from build123d import *

# Parameters (mm, degrees)
CROQUIS1_W                        = 25
CROQUIS1_H                        = 12.5
CROQUIS2_R                        = 3.5
SALIENTE_EXTRUIR1_DEPTH           = 2.5
CROQUIS3_R                        = 1.75
SALIENTE_EXTRUIR2_DEPTH           = 9.5
CORTAR_EXTRUIR1_DEPTH             = 8
CROQUIS5_R                        = 12.2
SALIENTE_EXTRUIR3_DEPTH           = 18
DI_METRO_DE_TALADRO_3_0_3_1_D     = 3
DI_METRO_DE_TALADRO_3_0_3_1_DEPTH = 8
CROQUIS10_R                       = 11.5
CORTAR_EXTRUIR2_DEPTH             = 2
SALIENTE_EXTRUIR4_DEPTH           = 1
CROQUIS12_W                       = 0.4
CROQUIS12_H                       = 3
SALIENTE_EXTRUIR5_DEPTH           = 6
REDONDEO1_R                       = 1
CORTAR_EXTRUIR3_DEPTH             = 57.252161552
CROQUIS15_R                       = 2.5
SALIENTE_EXTRUIR6_DEPTH           = 2
CROQUIS16_R                       = 1.5
SALIENTE_EXTRUIR7_DEPTH           = 3
CHAFL_N1_SIZE2                    = 0.363970234
CHAFL_N1_SIZE                     = 1
CROQUIS17_R                       = 1
CORTAR_EXTRUIR4_DEPTH             = 1


with BuildPart() as part:
    # Croquis1 → Revolución1 (revolve)
    with BuildSketch(Plane(origin=(0, 0, 0), x_dir=(-1, 0, 0), z_dir=(0, 0, -1)), mode=Mode.PRIVATE) as revoluci_n1_sk:
        with Locations((14, 12.15)):
            Rectangle(CROQUIS1_W, CROQUIS1_H)
    revolve(revoluci_n1_sk.sketch.rotate(Axis((-1.5, 5.9, 0), (-1, 0, 0)), 270), axis=Axis((-1.5, 5.9, 0), (-1, 0, 0)))

    # Croquis2 → Saliente-Extruir1 (add)
    with BuildSketch(Plane(origin=(-1.5, 0, 0), x_dir=(0, 0, -1), z_dir=(1, 0, 0))):
        with Locations((0, 5.9)):
            Circle(CROQUIS2_R)
    extrude(amount=SALIENTE_EXTRUIR1_DEPTH)

    # Croquis3 → Saliente-Extruir2 (add)
    with BuildSketch(Plane(origin=(1, 0, 0), x_dir=(0, 0, -1), z_dir=(1, 0, 0))):
        with Locations((0, 5.9)):
            Circle(CROQUIS3_R)
    extrude(amount=SALIENTE_EXTRUIR2_DEPTH)

    # Croquis4 → Cortar-Extruir1 (cut)
    with BuildSketch(Plane(origin=(10.5, 0, 0), x_dir=(0, 0, -1), z_dir=(1, 0, 0))):
        with BuildLine():
            Line((-1.496663044, 4.15), (1.496663044, 4.15))
            ThreePointArc((1.496663044, 4.15), (0, 4.264202971), (-1.496663044, 4.15))
        make_face()
    extrude(amount=-CORTAR_EXTRUIR1_DEPTH, mode=Mode.SUBTRACT)

    # Croquis5 → Saliente-Extruir3 (add)
    with BuildSketch(Plane.ZY.offset(26.5)):
        with Locations((0, 5.9)):
            Circle(CROQUIS5_R)
    extrude(amount=SALIENTE_EXTRUIR3_DEPTH)

    # Diámetro de taladro Ø3.0 (3)1
    with Locations(Plane(origin=(-1.5, 0, 0), x_dir=(0, 0, -1), z_dir=(1, 0, 0))):
        with Locations((-8.5, 5.827133015), (8.5, 5.827133015)):
            Hole(DI_METRO_DE_TALADRO_3_0_3_1_D / 2, depth=DI_METRO_DE_TALADRO_3_0_3_1_DEPTH)

    # Croquis10 → Cortar-Extruir2 (cut)
    with BuildSketch(Plane.ZY.offset(44.5)):
        with Locations((0, 5.9)):
            Circle(CROQUIS10_R)
    extrude(amount=-CORTAR_EXTRUIR2_DEPTH, mode=Mode.SUBTRACT)

    # Croquis11 → Saliente-Extruir4 (add)
    with BuildSketch(Plane.ZY.offset(42.5)):
        with BuildLine():
            Line((-5.135046812, 3.4), (-6.135046812, 3.4))
            ThreePointArc((-6.135046812, 3.4), (-6.488600202, 3.546446609), (-6.635046812, 3.9))
            Line((-6.635046812, 3.9), (-6.635046812, 7.9))
            ThreePointArc((-6.635046812, 7.9), (-6.488600202, 8.253553391), (-6.135046812, 8.4))
            Line((-6.135046812, 8.4), (-5.135046812, 8.4))
            ThreePointArc((-5.135046812, 8.4), (-4.781493421, 8.253553391), (-4.635046812, 7.9))
            Line((-4.635046812, 7.9), (-4.635046812, 3.9))
            ThreePointArc((-4.635046812, 3.9), (-4.781493421, 3.546446609), (-5.135046812, 3.4))
        make_face()
        with BuildLine():
            Line((7.124953188, 3.4), (6.124953188, 3.4))
            ThreePointArc((6.124953188, 3.4), (5.771399798, 3.546446609), (5.624953188, 3.9))
            Line((5.624953188, 3.9), (5.624953188, 7.9))
            ThreePointArc((5.624953188, 7.9), (5.771399798, 8.253553391), (6.124953188, 8.4))
            Line((6.124953188, 8.4), (7.124953188, 8.4))
            ThreePointArc((7.124953188, 8.4), (7.478506579, 8.253553391), (7.624953188, 7.9))
            Line((7.624953188, 7.9), (7.624953188, 3.9))
            ThreePointArc((7.624953188, 3.9), (7.478506579, 3.546446609), (7.124953188, 3.4))
        make_face()
    extrude(amount=SALIENTE_EXTRUIR4_DEPTH)

    # Croquis12 → Saliente-Extruir5 (add)
    with BuildSketch(Plane.ZY.offset(43.5)):
        with Locations((-5.637636684, 5.837666005)):
            Rectangle(CROQUIS12_W, CROQUIS12_H)
        with Locations((6.677710889, 5.9)):
            Rectangle(CROQUIS12_W, CROQUIS12_H)
    extrude(amount=SALIENTE_EXTRUIR5_DEPTH)

    # Redondeo1
    redondeo1_edges = [part.edges().sort_by_distance(p)[0] for p in [
        (-49.5, 4.337666005, -5.637636684),
        (-49.5, 7.337666005, -5.637636684),
        (-49.5, 4.4, 6.677710889),
        (-49.5, 7.4, 6.677710889),
    ]]
    fillet(redondeo1_edges, radius=REDONDEO1_R)

    # Croquis14 → Cortar-Extruir3 (cut, through all)
    with BuildSketch(Plane.XY.offset(6.877710889)):
        with BuildLine():
            Line((-45.3, 5.2), (-47.7, 5.2))
            ThreePointArc((-47.7, 5.2), (-47.912132034, 5.287867966), (-48, 5.5))
            Line((-48, 5.5), (-48, 6.3))
            ThreePointArc((-48, 6.3), (-47.912132034, 6.512132034), (-47.7, 6.6))
            Line((-47.7, 6.6), (-45.3, 6.6))
            ThreePointArc((-45.3, 6.6), (-45.087867966, 6.512132034), (-45, 6.3))
            Line((-45, 6.3), (-45, 5.5))
            ThreePointArc((-45, 5.5), (-45.087867966, 5.287867966), (-45.3, 5.2))
        make_face()
    extrude(amount=-CORTAR_EXTRUIR3_DEPTH, mode=Mode.SUBTRACT)

    # Croquis15 → Saliente-Extruir6 (add)
    with BuildSketch(Plane.ZY.offset(42.5)):
        with Locations((0, 5.9)):
            Circle(CROQUIS15_R)
    extrude(amount=SALIENTE_EXTRUIR6_DEPTH)

    # Croquis16 → Saliente-Extruir7 (add)
    with BuildSketch(Plane.ZY.offset(42.5)):
        with Locations((0, 5.9)):
            Circle(CROQUIS16_R)
    extrude(amount=SALIENTE_EXTRUIR7_DEPTH)

    # Chaflán1
    chafl_n1_edges = [part.edges().sort_by_distance(p)[0] for p in [
        (-45.5, 5.9, -1.5),
    ]]
    chafl_n1_side = [part.faces().sort_by_distance(p)[0] for p in [
        (-45.492720595, 5.9, -1.5),
    ]]
    chamfer(chafl_n1_edges, length=CHAFL_N1_SIZE - 0.0001, length2=CHAFL_N1_SIZE2 - 0.0001, reference=chafl_n1_side[0])  # a hair under: the kernel refuses the full size

    # Croquis17 → Cortar-Extruir4 (cut)
    with BuildSketch(Plane.ZY.offset(45.5)):
        with Locations((0, 5.9)):
            Circle(CROQUIS17_R)
    extrude(amount=-CORTAR_EXTRUIR4_DEPTH, mode=Mode.SUBTRACT)


solid = part.part
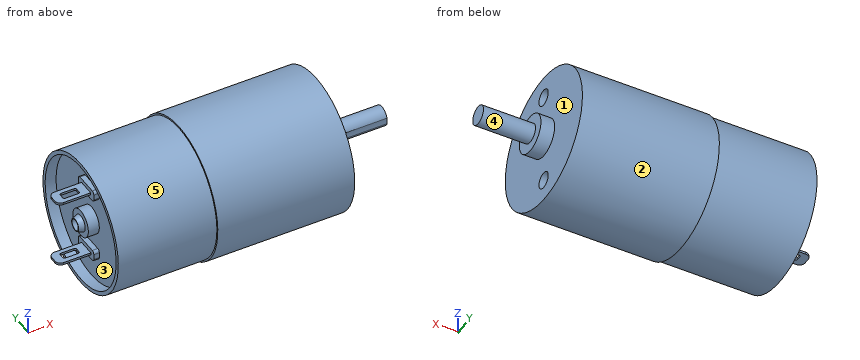
The model under review builds one solid part; all positions refer to its coordinate system, in mm. Face numbers are marked on the shaded views. A direction names the side the tool comes from. Coordinates: 2 decimals unless noted, no trailing zeros. Write each loop counter-clockwise with the first axis right and the second up, starting at its lowest first coordinate (ties: lowest second). Pieces come first, ordered by that corner, then holes. Notation, with made-up numbers: M 50,35.25 L 94,35.25 A16 cw 94,49.25 Z; hole C -26.5,-7 d9. An arc over 180 degrees is marked long. Put each result on its own line as item: value.
1) Add section B-B on z = 4.5. Give the boundary of the cut face in (x, y), then the cut area to 3 significant figures.
Computed:
outline: M -44.5,-5.44 L -26.5,-5.44 L -26.5,-5.76 L -1.5,-5.76 L -1.5,17.56 L -26.5,17.56 L -26.5,17.24 L -44.5,17.24 L -44.5,16.48 L -42.5,16.48 L -42.5,-4.68 L -44.5,-4.68 Z
area: 949 mm2
2) Draft analysis for pull direction Z (two halves, no side actions). For the marked faces 1, 2 and 3, state which applies: released by +Z, released by -Z, zero draft, split by the parting line, or undercut.
Computed:
face 1: zero draft
face 2: split by the parting line
face 3: undercut
3) Clearance check with flat-ended pins moving along their axes: pin 1 Ø8 at (x, z) = (-36, -5) entering from -Y; pin 2 Ø6 at (y, z) = (9.5, 8.5) entering from -X; pin 3 Ø8 at (x, z) = (-25, -9) entering from +Y. State where each tip first meets the part, or that it passes through.
Computed:
pin 1: stops at y = -6.26
pin 2: stops at x = -49.32
pin 3: stops at y = 17.36
4) Add section C-C on x = -40.5. Give the boundary of the cut face in (y, z), then the cut area to 3 significant figures.
Computed:
outline: C 5.9,0 d24.4
area: 468 mm2
5) Add section A-A on y = -1.5. Give the boundary of the cut face in (x, z), then the cut area to 3 significant figures.
Computed:
outline: M -44.5,-9.7 L -26.5,-9.7 L -26.5,-10.07 L -1.5,-10.07 L -1.5,10.07 L -26.5,10.07 L -26.5,9.7 L -44.5,9.7 L -44.5,8.8 L -42.5,8.8 L -42.5,-8.8 L -44.5,-8.8 Z
area: 818 mm2
6) Wall thickness on probe 1 along Z at (x, y) = (-30.5, 6.25); probe 2 along X at (y, z) = (-1.5, 7.25); probe 3 along Y at (x, z) = (-43.5, 9.5): over which ranges is each line inside the solid? List them lowest first. Write a range as [from, to].
Computed:
probe 1: z = [-12.19, 12.19]
probe 2: x = [-42.5, -1.5]
probe 3: y = [-1.75, -0.58], [12.38, 13.55]
7) Add section D-D on x = -5. Give the boundary of the cut face in (y, z).
Computed:
outline: C 5.9,0 d25; hole C 5.83,-8.5 d3; hole C 5.83,8.5 d3
8) For the marked faces 4 and 5, list the 3-axis set-ups (+Z, -Z, +X, -X, +Y, -Y) from which the entire face can be reached by the end or side of a thin tool; tool diameter is ignored.
Computed:
face 4: +X
face 5: -X
